Check sheet for the modelled part. Datum: model origin and axes. Units: mm. A direction names the side the tool comes from. Give positions to 0.01 mm unless a question says otherwise; leave off trailing zeros. Order: outer loops, then holes, each group sorted by start corner. A loop starts at its lowest first (then second) coordinate and runs counter-clockwise, first axis right, second up. Notation, with made-up numbers: (43.5, -22) - (81.5, -22) arc R14 cw to (81.5, -5) - close; hole circle Ø2 at (38.25, 42). An arc over 180 degrees is marked (long way). Answer in a Markdown table with one row per item.
Autodesk Inventor part; units mm, degrees
ref_plane "YZ Plane" through (0, 0, 0) normal (1, 0, 0) x (0, 1, 0)
ref_plane "XZ Plane" through (0, 0, 0) normal (0, 1, 0) x (-1, 0, 0)
ref_plane "XY Plane" through (0, 0, 0) normal (0, 0, 1) x (1, 0, 0)
sketch "Sketch1" plane through (0, 0, 0) normal (0, 1, 0) x (-1, 0, 0)
  line L0 (-40, 0) -> (-40, -100)
  line L1 (0, -100) -> (0, 0)
  line L2 (-35, 0) -> (-35, -100)
  line L3 (-6, -100) -> (-6, 0)
  circle A0 centre (-2.5, -50) radius 1.65
  circle A1 centre (-37.5, -50) radius 1.65
  line L4 (0, 0) -> (-8.5, 0)
  line L5 (-32.5, 0) -> (-40, 0)
  line L6 (-40, -100) -> (-32.5, -100)
  line L7 (-8.5, -100) -> (0, -100)
  line L8 (-8.5, 0) -> (-8.5, -100)
  line L9 (-32.5, -100) -> (-32.5, 0)
  dimension "d4" = 3.3
  dimension "d5" = 3.3
  dimension "d8" = 2.5
  dimension "d9" = 2.5
extrude "Extrusion1" add sketch "Sketch1" along normal blind 3.5
sketch "Sketch2" plane through (0, 3.5, 0) normal (0, 1, 0) x (1, 0, 0)
  line L0 (8.5, 100) -> (0, 100)
  line L1 (8.5, 100) -> (6, 100)
  line L2 (6, 100) -> (6, 0)
  line L3 (6, 0) -> (8.5, 0)
  line L4 (8.5, 0) -> (8.5, 100)
  line L5 (32.5, 100) -> (32.5, 0)
  line L6 (32.5, 100) -> (35, 100)
  line L7 (35, 100) -> (35, 0)
  line L8 (35, 0) -> (32.5, 0)
  line L9 (32.5, 0) -> (32.5, 100)
  point P0 (0, 0)
  point P1 (32.5, 0)
  point P2 (6, 100)
  dimension "d10" = 2.5
  dimension "d11" = 100
  dimension "d12" = 2.5
  dimension "d13" = 100
extrude "Extrusion2" add sketch "Sketch2" along normal blind 20
sketch "Sketch3" plane through (0, 23.5, 0) normal (0, 1, 0) x (1, 0, 0)
  line L0 (6, 100) -> (6, 0)
  line L1 (35, 100) -> (35, 0)
  line L2 (6, 0) -> (35, 0)
  line L3 (35, 0) -> (35, 100)
  line L4 (35, 100) -> (6, 100)
  line L5 (6, 100) -> (6, 0)
  point P0 (0, 0)
  point P1 (35, 0)
  point P2 (6, 100)
extrude "Extrusion3" add sketch "Sketch3" along normal blind 3.5
sketch "Sketch4" plane through (0, 27, 0) normal (0, 1, 0) x (1, 0, 0)
  circle A0 centre (9.75, 80.75) radius 1.15
  circle A1 centre (30.25, 80.75) radius 1.15
  circle A2 centre (9.75, 19.25) radius 1.15
  circle A3 centre (30.25, 19.25) radius 1.15
  line L0 (15.5, 70) -> (25.5, 70)
  line L1 (25.5, 70) -> (25.5, 30)
  line L2 (25.5, 30) -> (15.5, 30)
  line L3 (15.5, 30) -> (15.5, 70)
  circle A4 centre (15.5, 70) radius 1.15
  circle A5 centre (25.5, 70) radius 1.15
  circle A6 centre (15.5, 30) radius 1.15
  circle A7 centre (25.5, 30) radius 1.15
  dimension "d29" = 10
  dimension "d30" = 40
extrude "Extrusion4" cut sketch "Sketch4" against normal blind 3.5 contours L3 A4 L0 | L0 A4 L3 | A5 L1 L0 | L0 L1 A5 | A6 L2 L3 | L3 L2 A6 | A7 L2 L1 | L1 L2 A7
fillet "Fillet1" radius 0.3 24 edges at (6, 15.25, -100) (3, 3.5, -100) (20.5, 27, -100) (8.5, 11.75, -100) (20.5, 23.5, -100) (35, 15.25, -100) (32.5, 11.75, -100) (32.5, 11.75, 0) (35, 15.25, 0) (20.5, 27, 0) (20.5, 23.5, 0) (8.5, 11.75, 0) (6, 15.25, 0) (6, 27, -50) (35, 27, -50) (0, 3.5, -50) (40, 3.5, -50) (37.5, 3.5, 0) (3, 3.5, 0) (0, 1.75, 0) (40, 1.75, 0) (40, 1.75, -100) (37.5, 3.5, -100) (0, 1.75, -100)
fillet "Fillet2" radius 0.3 6 edges at (6.0879, 3.4121, -99.9121) (6.0879, 3.4121, -0.0879) (6, 3.5, -50) (34.9121, 3.4121, -0.0879) (34.9121, 3.4121, -99.9121) (35, 3.5, -50)
properties part number "controllerHousing"
(1) Gauge pin test, flat ends, axial feed: P1, Ø7, axis at y = 8, z = -47, coming from the -X side; P2, Ø12, axis at x = 22, z = -42.5, coming from the -Y side; P3, Ø2.5, axis at x = 4, z = -67, coming from the +Y side. Record the tip position at first contact, or that the pin passes through.
Geometry says:
| item | result |
|---|---|
| P1 | x = 6 |
| P2 | y = 23.5 |
| P3 | y = 3.5 |
(2) Cross-section at D-D, the plane x = 15.5. Record the cut outline in (y, z).
Geometry says:
| item | result |
|---|---|
| outline | (23.5, -99.7) arc R0.3 ccw to (23.8, -100) - (26.7, -100) arc R0.3 ccw to (27, -99.7) - (27, -71.15) - (23.5, -71.15) - close; (23.5, -68.85) - (27, -68.85) - (27, -31.15) - (23.5, -31.15) - close; (23.5, -28.85) - (27, -28.85) - (27, -0.3) arc R0.3 ccw to (26.7, 0) - (23.8, 0) arc R0.3 ccw to (23.5, -0.3) - close |
(3) Cross-section at A-A, the plane z = -70. Record the cut outline in (x, y).
Geometry says:
| item | result |
|---|---|
| outline | (0, 0) - (8.5, 0) - (8.5, 23.5) - (14.35, 23.5) - (14.35, 27) - (6.3, 27) arc R0.3 ccw to (6, 26.7) - (6, 3.8) arc R0.3 cw to (5.7, 3.5) - (0.3, 3.5) arc R0.3 ccw to (0, 3.2) - close; (16.65, 23.5) - (24.35, 23.5) - (24.35, 27) - (16.65, 27) - close; (26.65, 23.5) - (32.5, 23.5) - (32.5, 0) - (40, 0) - (40, 3.2) arc R0.3 ccw to (39.7, 3.5) - (35.3, 3.5) arc R0.3 cw to (35, 3.8) - (35, 26.7) arc R0.3 ccw to (34.7, 27) - (26.65, 27) - close |
(4) Mould release check, pull along X, two halves, no side actions. Record for faces 5 (the flat face through (21, 24, 0)), 6 (the flat face through (0, 2, -51)), 7 (the flat face through (20, 23.5, -51)): pulls with the +X half, pulls with the -X half, needs draft (parallel to the pull), parting line crosses it, or undercut.
Geometry says:
| item | result |
|---|---|
| face 5 | needs draft |
| face 6 | pulls with the -X half |
| face 7 | undercut |
(5) Thickness scan on L1, parallel to X at y = 25.65, z = -30; L2, parallel to Z at x = 25.5, y = 26.35; L3, parallel to X at y = 4.25, z = -93. Record the ranges inside material, lowest first.
Geometry says:
| item | result |
|---|---|
| L1 | 6 to 14.35, 16.65 to 24.35, 26.65 to 35 |
| L2 | -100 to -71.15, -68.85 to -31.15, -28.85 to 0 |
| L3 | 6 to 8.5, 32.5 to 35 |
(6) Access from +Z, -Z, +X, -X, +Y, -Y to the whole of each face (thin tool, end or side, straight path). Record for faces 1 (the cylindrical face through (15.251, 25.274, -28.877)), 2 (the flat face through (6, 15, -51)), 3 (the flat face through (35, 15, -51)), 4 (the flat face through (32.5, 12, -51)).
Geometry says:
| item | result |
|---|---|
| face 1 | +Y, -Y |
| face 2 | +Z, -Z, -X, +Y |
| face 3 | +Z, -Z, +X, +Y |
| face 4 | +Z, -Z, -Y |
(7) Cross-section at B-B, the plane x = 2.5. Record the cut outline in (y, z), then the cut area to 3 significant figures.
Geometry says:
| item | result |
|---|---|
| outline | (0, -100) - (3.2, -100) arc R0.3 ccw to (3.5, -99.7) - (3.5, -51.65) - (0, -51.65) - close; (0, -48.35) - (3.5, -48.35) - (3.5, -0.3) arc R0.3 ccw to (3.2, 0) - (0, 0) - close |
| area | 338 mm² |
(8) Cross-section at C-C, the plane y = 7. Record the cut outline in (x, z), then the cut area to 3 significant figures.
Geometry says:
| item | result |
|---|---|
| outline | (6, -99.7) arc R0.3 ccw to (6.3, -100) - (8.2, -100) arc R0.3 ccw to (8.5, -99.7) - (8.5, -0.3) arc R0.3 ccw to (8.2, 0) - (6.3, 0) arc R0.3 ccw to (6, -0.3) - close; (32.5, -99.7) arc R0.3 ccw to (32.8, -100) - (34.7, -100) arc R0.3 ccw to (35, -99.7) - (35, -0.3) arc R0.3 ccw to (34.7, 0) - (32.8, 0) arc R0.3 ccw to (32.5, -0.3) - close |
| area | 500 mm² |
